from build123d import *

# Parameters (mm, degrees)
SKETCH1_R           = 5.75
SKETCH1_R_2         = 1.65
BOSS_EXTRUDE1_DEPTH = 10
SKETCH2_R           = 2
BOSS_EXTRUDE2_DEPTH = 4
FILLET1_R           = 2


with BuildPart() as part:
    # Sketch1 → Boss-Extrude1 (new body)
    with BuildSketch(Plane(origin=(0, 0, 0), x_dir=(1, 0, 0), z_dir=(0, 1, 0))):
        with Locations(Location((0, 0, 0), (0, 0, 270))):
            Circle(SKETCH1_R)
        with Locations(Location((0, 0, 0), (0, 0, 270))):
            Circle(SKETCH1_R_2, mode=Mode.SUBTRACT)
    extrude(amount=BOSS_EXTRUDE1_DEPTH)

    # Sketch2 → Boss-Extrude2 (add)
    # profile 1 of 4: a face of its own
    with BuildSketch(Plane.XZ):
        with BuildLine():
            ThreePointArc((20.75, 0), (19.065863992, 4.065863992), (15, 5.75))
            Line((15, 5.75), (9.25, 0))
            Line((9.25, 0), (15, -5.75))
            ThreePointArc((15, -5.75), (19.065863992, -4.065863992), (20.75, 0))
        make_face()
        with Locations(Location((15, 0, 0), (0, 0, 270))):
            Circle(SKETCH2_R, mode=Mode.SUBTRACT)
    # profile 2 of 4: a face of its own
    with BuildSketch(Plane.XZ):
        with BuildLine():
            Line((9.25, 0), (15, 5.75))
            ThreePointArc((15, 5.75), (10.934136008, 4.065863992), (9.25, 0))
        make_face()
    # profile 3 of 4: a face of its own
    with BuildSketch(Plane.XZ):
        with BuildLine():
            ThreePointArc((9.25, 0), (10.934136008, 4.065863992), (15, 5.75))
            Line((15, 5.75), (0, 5.75))
            ThreePointArc((0, 5.75), (4.065863992, 4.065863992), (5.75, 0))
            ThreePointArc((5.75, 0), (4.065863992, -4.065863992), (0, -5.75))
            Line((0, -5.75), (15, -5.75))
            ThreePointArc((15, -5.75), (10.934136008, -4.065863992), (9.25, 0))
        make_face()
    # profile 4 of 4: a face of its own
    with BuildSketch(Plane.XZ):
        with BuildLine():
            Line((15, -5.75), (9.25, 0))
            ThreePointArc((9.25, 0), (10.934136008, -4.065863992), (15, -5.75))
        make_face()
    extrude(amount=-BOSS_EXTRUDE2_DEPTH)

    # Fillet1
    # the kernel refuses this fillet: 2 mm, written as the material it takes off along each edge
    with BuildSketch(Plane(origin=(-5, 4, -5.75), x_dir=(0, 0, 1), z_dir=(1, 0, 0))) as fillet1_piece_1_section:
        with BuildLine():
            CenterArc((FILLET1_R, FILLET1_R), FILLET1_R, 180, 90)
            Line((0, FILLET1_R), (0, 0))
            Line((0, 0), (FILLET1_R, 0))
        make_face()
    fillet1_piece_1 = extrude(amount=20, mode=Mode.PRIVATE)
    fillet1_piece_1 = fillet1_piece_1 - Plane(origin=(0, 3.514129047, 0), x_dir=(0, 0, 1), z_dir=(0, -1, 0)) * Cylinder(5.75, 48, mode=Mode.PRIVATE)
    add(fillet1_piece_1, mode=Mode.SUBTRACT)
    with BuildSketch(Plane(origin=(15, 4, 5.75), x_dir=(0, -1, 0), z_dir=(-1, 0, 0))) as fillet1_piece_2_section:
        with BuildLine():
            CenterArc((FILLET1_R, -FILLET1_R), FILLET1_R, 90, 90)
            Line((0, -FILLET1_R), (0, 0))
            Line((0, 0), (FILLET1_R, 0))
        make_face()
    fillet1_piece_2 = extrude(amount=20, mode=Mode.PRIVATE)
    fillet1_piece_2 = fillet1_piece_2 - Plane(origin=(0, 3.514130378, 0), x_dir=(0, 0, 1), z_dir=(0, -1, 0)) * Cylinder(5.75, 48, mode=Mode.PRIVATE)
    add(fillet1_piece_2, mode=Mode.SUBTRACT)
    with BuildSketch(Plane(origin=(15, 4, 0), x_dir=(0, 0, -1), z_dir=(-1, 0, 0))) as fillet1_piece_3:
        with BuildLine():
            CenterArc((5.75 - FILLET1_R, FILLET1_R), FILLET1_R, 270, 90)
            Line((5.75, FILLET1_R), (5.75, 0))
            Line((5.75, 0), (5.75 - FILLET1_R, 0))
        make_face()
    revolve(axis=Axis((15, 4, 0), (0, -1, 0)), revolution_arc=180, mode=Mode.SUBTRACT)


solid = part.part
Design review of the part built by this model. Coordinates are the model's own, in mm. A direction names the side the tool comes from. Give positions to 0.01 mm unless a question says otherwise; leave off trailing zeros. Order: outer loops, then holes, each group sorted by start corner. A loop starts at its lowest first (then second) coordinate and runs counter-clockwise, first axis right, second up.
1. Add section A-A, the plane y = 1.5. State the section outline as (x, z) points, then the cut area to 3 significant figures.
Solution:
outline: (0, -5.75) - (15, -5.75) arc R5.75 ccw to (15, 5.75) - (0, 5.75) arc R5.75 ccw to start; hole circle Ø3.3 at (0, 0); hole circle Ø4 at (15, 0)
area: 255 mm2
2. Mouldability with a two-part tool opening along X and no side actions: class faces 1 (the cylindrical face through (9.27, 3.4, 5.18)), 2 (the cylindrical face through (-5.613, 6.041, -1.246)), 3 (the cylindrical face through (-1, 4.93, -1.31)) as +X half, -X half, draft (parallel to the pull), parting line (faces both ways), or undercut.
Solution:
face 1: draft
face 2: parting line
face 3: undercut
3. Tool access review of faces 4 (the cylindrical face through (9.06, 3.4, -5.18)), 5 (the flat face through (1.4, 10, 1.2)): name each direction out of +Z, -Z, +X, -X, +Y, -Y from which nothing blocks a thin tool from reaching the whole face with its end or side.
Solution:
face 4: -Z, +X, +Y
face 5: +Z, -Z, +X, -X, +Y
4. Add section B-B, the plane x = 1. State the section outline as (y, z) points.
Solution:
outline: (0, -5.75) - (2, -5.75) arc R2 ccw to (2.59, -5.66) - (10, -5.66) - (10, -1.31) - (0, -1.31) - close; (0, 1.31) - (10, 1.31) - (10, 5.66) - (2.59, 5.66) arc R2 ccw to (2, 5.75) - (0, 5.75) - close
5. Add section C-C, the plane y = 7.75. State the section outline as (x, z) points, then the cut area to 3 significant figures.
Solution:
outline: circle Ø11.5 at (0, 0); hole circle Ø3.3 at (0, 0)
area: 95.3 mm2
6. To check wall thickness, follow L1, parallel to X at y = 6.25, z = 0; L2, parallel to X at y = 3, z = 0.25; L3, parallel to X at y = 1.25, z = -1.5. State the ranges of each line that lie inside material, in increasing order.
Solution:
L1: x = -5.75 to -1.65, 1.65 to 5.75
L2: x = -5.74 to -1.63, 1.63 to 13.02, 16.98 to 20.48
L3: x = -5.55 to -0.69, 0.69 to 13.68, 16.32 to 20.55
7. For pin 1 Ø6 at (x, z) = (9, -1) entering from +Y; pin 2 Ø5.5 at (x, z) = (0, 0) entering from -Y; pin 3 Ø3 at (y, z) = (6, -0.5) entering from +X; pin 4 Ø1 at (x, y) = (-1.5, 4) entering from -Z, all flat-tipped, find the tip position at first contact; note any pin that passes through.
Solution:
pin 1: stops at y = 4
pin 2: stops at y = 0
pin 3: stops at x = 5.75
pin 4: stops at z = -5.66
8. Add section D-D, the plane x = 12. State the section outline as (y, z) points, then the cut area to 3 significant figures.
Solution:
outline: (0, -5.75) - (2, -5.75) arc R2 ccw to (4, -3.75) - (4, 3.75) arc R2 ccw to (2, 5.75) - (0, 5.75) - close
area: 44.3 mm2
